Check sheet for the drawn part. Datum: minimum x, y, z corner. Units: mm. Round coordinates to 2 decimals unless told otherwise and drop trailing zeros. Write each loop counter-clockwise with the first axis right and the second up, starting at its lowest first coordinate (ties: lowest second). Pieces come first, ordered by that corner, then holes. Notation, with made-up numbers: M 62,18 L 114,18 A17 ccw 114,34 Z; hole C 31.25,-20.75 d5. An arc over 180 degrees is marked long. Put each result on its own line as item: value.
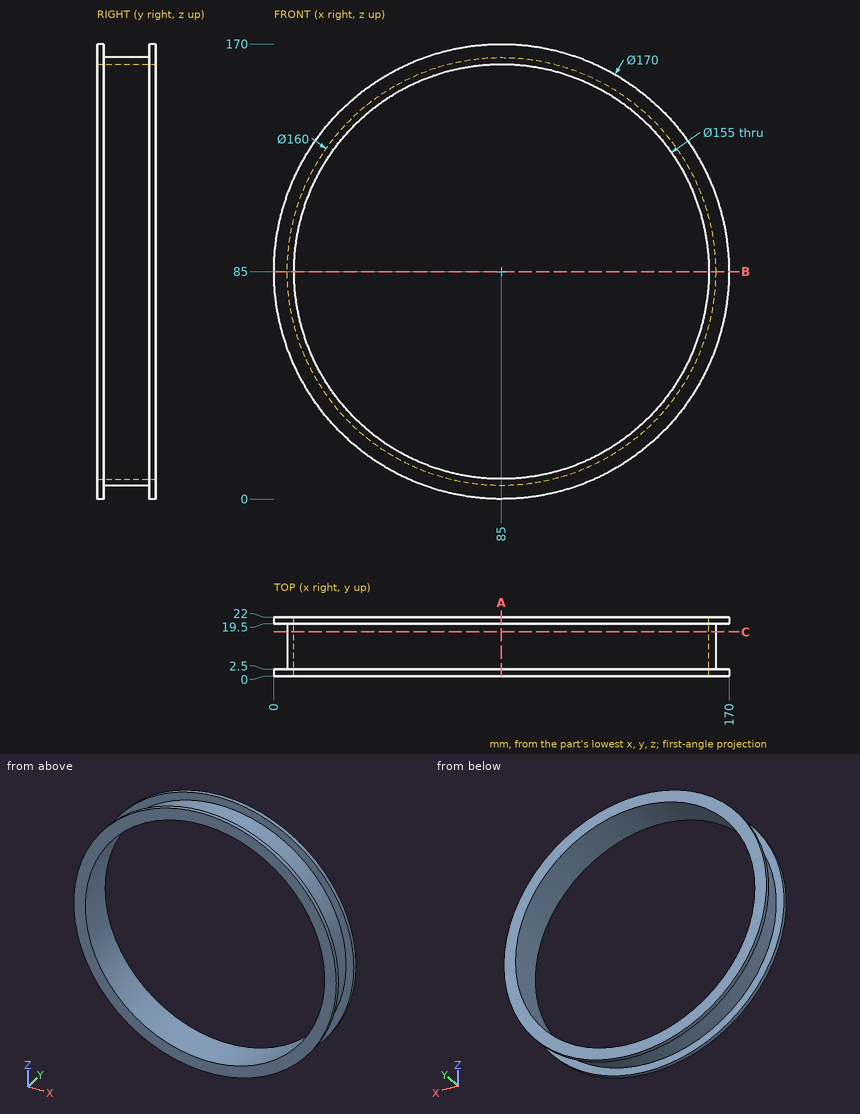
1. Cross-section at A-A (x = 85). Enter the section's corners in (y, z), then the cut area to 3 significant figures.
Computed values:
outline: M 0,0 L 2.5,0 L 2.5,5 L 19.5,5 L 19.5,0 L 22,0 L 22,7.5 L 0,7.5 Z; M 0,162.5 L 22,162.5 L 22,170 L 19.5,170 L 19.5,165 L 2.5,165 L 2.5,170 L 0,170 Z
area: 160 mm2
2. Cross-section at C-C (y = 16.5). Enter the section's corners in (x, z), then the cut area to 3 significant figures.
Computed values:
outline: C 85,85 d160; hole C 85,85 d155
area: 1,240 mm2
3. Depth check by flat-ended pin: pin 1 Ø12 at (x, y) = (142.5, 7) entering from +Z; pin 2 Ø10 at (y, z) = (10.5, 144.5) entering from +X; pin 3 Ø3 at (y, z) = (4.5, 136.5) entering from -X. Enter the tip coordinate at first touch or a pass-through.
Computed values:
pin 1: stops at z = 151.03
pin 2: stops at x = 143.56
pin 3: stops at x = 22.55
4. Cross-section at B-B (z = 85). Enter the section's corners in (x, y), then the cut area to 3 significant figures.
Computed values:
outline: M 0,0 L 7.5,0 L 7.5,22 L 0,22 L 0,19.5 L 5,19.5 L 5,2.5 L 0,2.5 Z; M 162.5,0 L 170,0 L 170,2.5 L 165,2.5 L 165,19.5 L 170,19.5 L 170,22 L 162.5,22 Z
area: 160 mm2
5. Scan lines: probe 1 along X at (y, z) = (19.75, 86.5); probe 2 along X at (y, z) = (8.5, 85). Record each from-to range of solid material in increasing order.
Computed values:
probe 1: x = 0.01 to 7.51, 162.49 to 169.99
probe 2: x = 5 to 7.5, 162.5 to 165
